Could you check a few things on this model? Use its own coordinates, in mm. Round coordinates to 2 decimals unless told otherwise and drop trailing zeros. Loops run counter-clockwise (first coordinate to the right, second up) from the corner with the lowest first, then second, coordinate; pieces in that order, holes last.
from build123d import *

# Parameters (mm, degrees)
SKETCH_1_R      = 1.25
SKETCH_1_R_2    = 1.500000002
SKETCH_1_W      = 22.999938461
SKETCH_1_H      = 12.000117949
SKETCH_1_W_2    = 2.999969231
SKETCH_1_H_2    = 6.000015385
SKETCH_1_W_3    = 9.999984615
SKETCH_1_H_3    = 3.000051282
SKETCH_1_W_4    = 10
SKETCH_1_H_4    = 6
SKETCH_1_W_5    = 9.999984616
EXTRUDE_1_DEPTH = 3


with BuildPart() as part:
    # 草圖1 → 填料-伸長1 (new body)
    with BuildSketch(Plane.XY):
        with BuildLine():
            Line((149.545923845, 145.649704894), (101.475469426, 154.53805141))
            ThreePointArc((101.475469426, 154.53805141), (99.077497598, 154.23914087), (97.289259558, 152.613772878))
            Line((97.289259558, 152.613772878), (92.406316445, 144.206797918))
            ThreePointArc((92.406316445, 144.206797918), (92.103687803, 143.480249781), (92.000408718, 142.7))
            Line((92.000408718, 142.7), (92.0003, 99))
            ThreePointArc((92.0003, 99), (92.878928766, 96.87870585), (95.000184615, 95.999984616))
            Line((95.000184615, 95.999984616), (149.000184614, 95.999707693))
            ThreePointArc((149.000184614, 95.999707693), (151.121568411, 96.878376105), (152.000399999, 98.999692307))
            Line((152.000399999, 98.999692307), (152.001144765, 143.013690924))
            ThreePointArc((152.001144765, 143.013690924), (151.188953144, 144.718624927), (149.545923845, 145.649704894))
        make_face()
        with Locations((131.500611289, 142.699797442)):
            Circle(SKETCH_1_R, mode=Mode.SUBTRACT)
        with Locations((147.500257437, 113.199715383)):
            Circle(SKETCH_1_R_2, mode=Mode.SUBTRACT)
        with Locations((122.000316411, 105.199794873)):
            Circle(SKETCH_1_R_2, mode=Mode.SUBTRACT)
        with Locations((100.748149255, 150.60475514)):
            Circle(SKETCH_1_R, mode=Mode.SUBTRACT)
        Polygon((102.176568231, 125.699947814), (99.176568231, 125.699963199), (99.176619513, 135.699963199), (102.176619513, 135.699947814), align=None, mode=Mode.SUBTRACT)
        with Locations((131.500362564, 133.699797435)):
            Rectangle(SKETCH_1_W, SKETCH_1_H, mode=Mode.SUBTRACT)
        with Locations((147.500290769, 119.699715384)):
            Rectangle(SKETCH_1_W_2, SKETCH_1_H_2, mode=Mode.SUBTRACT)
        with Locations((139.50021641, 105.19975641)):
            Rectangle(SKETCH_1_W_3, SKETCH_1_H_3, mode=Mode.SUBTRACT)
        with Locations((147.500224102, 106.699715384)):
            Rectangle(SKETCH_1_W_2, SKETCH_1_H_2, mode=Mode.SUBTRACT)
        with Locations((114.500224102, 111.699910257)):
            Rectangle(SKETCH_1_W_4, SKETCH_1_H_4, mode=Mode.SUBTRACT)
        with Locations((104.50021641, 105.199935898)):
            Rectangle(SKETCH_1_W_5, SKETCH_1_H_3, mode=Mode.SUBTRACT)
    extrude(amount=EXTRUDE_1_DEPTH)


solid = part.part
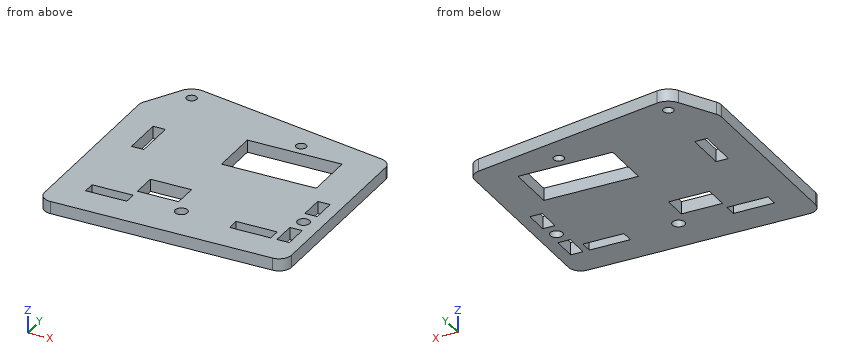
Item 1: If we section it at B-B, the plane y = 121.5: Please give me the cut outline in (x, z).
Results list:
outline: (92, 0) - (146, 0) - (146, 3) - (92, 3) - close; (149, 0) - (152, 0) - (152, 3) - (149, 3) - close
Item 2: If we section it at D-D, the plane z = 0.9: Count the separate pieces of the cut face and the enclosed holes in it, then the cut area to 3 significant figures.
Results list:
separate pieces: 1
enclosed holes: 11
area: 2,750 mm2
Item 3: If we section it at C-C, the plane y = 130: Please give me the cut outline in (x, z).
Results list:
outline: (92, 0) - (99.18, 0) - (99.18, 3) - (92, 3) - close; (102.18, 0) - (120, 0) - (120, 3) - (102.18, 3) - close; (143, 0) - (152, 0) - (152, 3) - (143, 3) - close
Item 4: If I drill on line 1 along X through (y, z) = (109, 2); line 2 along X through (y, z) = (129.5, 2.6); line 3 along X through (y, z) = (104.5, 2.4), over which ranges is the centre line in solid material (lowest first)?
Results list:
line 1: x = 92 to 109.5, 119.5 to 146, 149 to 152
line 2: x = 92 to 99.18, 102.18 to 120, 143 to 152
line 3: x = 92 to 99.5, 109.5 to 120.67, 123.33 to 134.5, 144.5 to 146, 149 to 152
Item 5: Will these pins go through, and if not, where does the flat tip stop? pin 1 (1.5 mm diameter, centred on x = 112.5, z = 2, fed in from +Y); pin 2 (1.5 mm diameter, centred on x = 104, z = 1.5, fed in from +Y).
Results list:
pin 1: stops at y = 152.64
pin 2: stops at y = 154.21
Item 6: If we section it at A-A, the plane x = 141: Please give me the cut outline in (y, z).
Results list:
outline: (96, 0) - (103.7, 0) - (103.7, 3) - (96, 3) - close; (106.7, 0) - (127.7, 0) - (127.7, 3) - (106.7, 3) - close; (139.7, 0) - (147.23, 0) - (147.23, 3) - (139.7, 3) - close
